from build123d import *

# Parameters (mm, degrees)
SALIENTE_EXTRUIR1_DEPTH = 5.5


with BuildPart() as part:
    # Croquis1 → Saliente-Extruir1 (new body)
    with BuildSketch(Plane(origin=(0, 0, 0), x_dir=(1, 0, 0), z_dir=(0, 1, 0))):
        Polygon((23, 3), (23, 0), (38, 0), (38, 3), (53, 3), (53, 0), (68, 0), (68, 3), (85.5, 3), (85.5, 13), (91, 13), (91, 33), (85.5, 33), (85.5, 53), (91, 53), (91, 73), (85.5, 73), (85.5, 93), (91, 93), (91, 113), (85.5, 113), (85.5, 133), (91, 133), (91, 153), (85.5, 153), (85.5, 166), (5.5, 166), (5.5, 153), (0, 153), (0, 133), (5.5, 133), (5.5, 113), (0, 113), (0, 93), (5.5, 93), (5.5, 73), (0, 73), (0, 53), (5.5, 53), (5.5, 33), (0, 33), (0, 13), (5.5, 13), (5.5, 3), align=None)
    extrude(amount=SALIENTE_EXTRUIR1_DEPTH)


solid = part.part
Verification items for the finished model (mm, model axes). A direction names the side the tool comes from. Give positions to 0.01 mm unless a question says otherwise; leave off trailing zeros. Loops run counter-clockwise (first coordinate to the right, second up) from the corner with the lowest first, then second, coordinate; pieces in that order, holes last. Notation, with made-up numbers: (29.5, 46) - (39.5, 46) arc R16 cw to (39.5, 68) - close; hole circle Ø11 at (50.25, -10.75). An arc over 180 degrees is marked (long way). Write each question's results on one line, items separated by ' | '.
1) Material ranges on L1, parallel to Z at x = 45, y = 2.1; L2, parallel to X at y = 2.15, z = -116, recorded low to high. Write a range as from..to.
Solution:
L1: -166..-3 | L2: 5.5..85.5
2) Tool access check on faces 5 (the flat face through (5.5, 3, -8)), 6 (the flat face through (85.5, 3, -8)), 7 (the flat face through (88, 3, -153)), 8 (the flat face through (5.5, 3, -123)), 9 (the flat face through (88, 3, -113)). Record the directions out of +Z, -Z, +X, -X, +Y, -Y that give a thin tool (end or side, any length) a straight path to the whole face; none if there is none.
Solution:
face 5: +Z, -X, +Y, -Y | face 6: +Z, +X, +Y, -Y | face 7: -Z, +X, +Y, -Y | face 8: -X, +Y, -Y | face 9: +X, +Y, -Y
3) Mould release check, pull along Z, two halves, no side actions. Record for faces 1 (the flat face through (85.5, 3, -123)), 2 (the flat face through (0, 3, -103)), 3 (the flat face through (3, 3, -73)), 4 (the flat face through (30, 3, 0)): pulls with the +Z half, pulls with the -Z half, needs draft (parallel to the pull), parting line crosses it, or undercut.
Solution:
face 1: undercut | face 2: needs draft | face 3: undercut | face 4: pulls with the +Z half
4) Sectioned sample at B-B on x = 19.5. Record the boundary of the cut face in (y, z), plus the area to 4 significant figures.
Solution:
outline: (0, -166) - (5.5, -166) - (5.5, -3) - (0, -3) - close | area: 896.5 mm2
5) Sectioned sample at A-A on z = -45. Record the boundary of the cut face in (x, y).
Solution:
outline: (5.5, 0) - (85.5, 0) - (85.5, 5.5) - (5.5, 5.5) - close
6) Depth check by flat-ended pin: P1, Ø1.6, axis at y = 2.5, z = -159, coming from the -X side; P2, Ø8, axis at x = 67.5, z = -124.5, coming from the -Y side; P3, Ø3, axis at y = 2, z = -41.5, coming from the +X side; P4, Ø1.5, axis at y = 3, z = -1, coming from the +X side. Enter the tip coordinate at first touch or a pass-through.
Solution:
P1: x = 5.5 | P2: y = 0 | P3: x = 85.5 | P4: x = 68
